```python
from build123d import *

# Parameters (mm, degrees)
HIERRO_ANGULAR_2_X_2_X_0_125_1_DEPTH = 150
CORTAR_EXTRUIR1_DEPTH                = 10
CORTAR_EXTRUIR2_REACH                = 168.317
CROQUIS4_R                           = 2.5


with BuildPart() as part:
    # Sketch1 → Hierro angular 2 X 2 X 0.125(1) (new body)
    with BuildSketch(Plane(origin=(0, 0, 0), x_dir=(1, 0, 0), z_dir=(0, 1, 0))):
        with BuildLine():
            Line((0, 0), (0, 50.8))
            Line((0, 50.8), (0.00508, 50.8))
            ThreePointArc((0.00508, 50.8), (2.246551928, 49.871551928), (3.175, 47.63008))
            Line((3.175, 47.63008), (3.175, 7.9375))
            ThreePointArc((3.175, 7.9375), (4.569903955, 4.569903955), (7.9375, 3.175))
            Line((7.9375, 3.175), (47.63008, 3.175))
            ThreePointArc((47.63008, 3.175), (49.871551928, 2.246551928), (50.8, 0.00508))
            Line((50.8, 0.00508), (50.8, 0))
            Line((50.8, 0), (0, 0))
        make_face()
    extrude(amount=HIERRO_ANGULAR_2_X_2_X_0_125_1_DEPTH)

    # Croquis3 → Cortar-Extruir1 (cut)
    with BuildSketch(Plane.XY):
        Polygon((25, 0), (50.8, 50), (50.8, 0), align=None)
    extrude(amount=-CORTAR_EXTRUIR1_DEPTH, mode=Mode.SUBTRACT)

    # Cortar-Extruir2: up to this face of the body (flat: up to its plane)
    cortar_extruir2_end = Plane(part.part.faces().sort_by_distance((26.665136317, 80.490198143, -3.175))[0])
    # Croquis4 → Cortar-Extruir2 (cut, up to the picked face)
    with BuildSketch(Plane.XY, mode=Mode.PRIVATE) as cortar_extruir2_sk1:
        with Locations((17.9, 140.12)):
            Circle(CROQUIS4_R)
    cortar_extruir2_tool1 = split(extrude(cortar_extruir2_sk1.sketch, amount=-CORTAR_EXTRUIR2_REACH, mode=Mode.PRIVATE), bisect_by=cortar_extruir2_end, keep=Keep.BOTH, mode=Mode.PRIVATE)
    # Croquis4 → Cortar-Extruir2 (cut, up to the picked face)
    with BuildSketch(Plane.XY, mode=Mode.PRIVATE) as cortar_extruir2_sk2:
        with Locations((45.4, 140.12)):
            Circle(CROQUIS4_R)
    cortar_extruir2_tool2 = split(extrude(cortar_extruir2_sk2.sketch, amount=-CORTAR_EXTRUIR2_REACH, mode=Mode.PRIVATE), bisect_by=cortar_extruir2_end, keep=Keep.BOTH, mode=Mode.PRIVATE)
    # Croquis4 → Cortar-Extruir2 (cut, up to the picked face)
    with BuildSketch(Plane.XY, mode=Mode.PRIVATE) as cortar_extruir2_sk3:
        with Locations((17.9, 59.87)):
            Circle(CROQUIS4_R)
    cortar_extruir2_tool3 = split(extrude(cortar_extruir2_sk3.sketch, amount=-CORTAR_EXTRUIR2_REACH, mode=Mode.PRIVATE), bisect_by=cortar_extruir2_end, keep=Keep.BOTH, mode=Mode.PRIVATE)
    # Croquis4 → Cortar-Extruir2 (cut, up to the picked face)
    with BuildSketch(Plane.XY, mode=Mode.PRIVATE) as cortar_extruir2_sk4:
        with Locations((45.4, 59.87)):
            Circle(CROQUIS4_R)
    cortar_extruir2_tool4 = split(extrude(cortar_extruir2_sk4.sketch, amount=-CORTAR_EXTRUIR2_REACH, mode=Mode.PRIVATE), bisect_by=cortar_extruir2_end, keep=Keep.BOTH, mode=Mode.PRIVATE)
    add(cortar_extruir2_tool1.solids().sort_by(Axis((17.9, 140.12, 0), (0, 0, -1)))[0], mode=Mode.SUBTRACT)
    add(cortar_extruir2_tool2.solids().sort_by(Axis((45.4, 140.12, 0), (0, 0, -1)))[0], mode=Mode.SUBTRACT)
    add(cortar_extruir2_tool3.solids().sort_by(Axis((17.9, 59.87, 0), (0, 0, -1)))[0], mode=Mode.SUBTRACT)
    add(cortar_extruir2_tool4.solids().sort_by(Axis((45.4, 59.87, 0), (0, 0, -1)))[0], mode=Mode.SUBTRACT)


solid = part.part
```
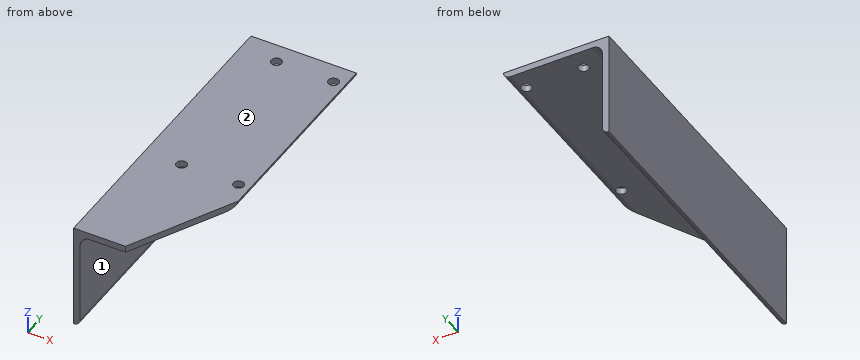
Work out the finished part from the listing and answer in its coordinate system (mm). Face numbers are marked on the shaded views. A direction names the side the tool comes from. Round coordinates to 2 decimals unless told otherwise and drop trailing zeros. Loops run counter-clockwise (first coordinate to the right, second up) from the corner with the lowest first, then second, coordinate; pieces in that order, holes last.
(1) For the marked faces 1 and 2, determine the directions among +Z, -Z, +X, -X, +Y, -Y from which every point of the face is accessible in a straight line to the end or side of a thin tool.
Computed values:
face 1: -Z, +X, +Y, -Y
face 2: +Z, +X, -X, +Y, -Y
(2) The part is cut by section A-A, the plane x = 17.9. Give the vertices of the cut face in (y, z) (3 decimals).
Computed values:
outline: (0, -3.175) - (57.37, -3.175) - (57.37, 0) - (0, 0) - close; (62.37, -3.175) - (137.62, -3.175) - (137.62, 0) - (62.37, 0) - close; (142.62, -3.175) - (150, -3.175) - (150, 0) - (142.62, 0) - close
(3) The part is cut by section D-D, the plane x = 45.4. Give the vertices of the cut face in (y, z) (3 decimals), and give its area (3 significant figures).
Computed values:
outline: (39.535, -3.175) - (57.37, -3.175) - (57.37, 0) - (39.535, 0) - close; (62.37, -3.175) - (137.62, -3.175) - (137.62, 0) - (62.37, 0) - close; (142.62, -3.175) - (150, -3.175) - (150, 0) - (142.62, 0) - close
area: 319 mm2
(4) Each of these flat-tipped pins is pushed along its axis until it touches: P1, Ø12, axis at x = 35, y = 59, coming from the -Z side (3 decimals); P2, Ø5, axis at y = 109, z = -27, coming from the +X side (3 decimals). Where does it stop, or does it pass through?
Computed values:
P1: stops at z = -3.175
P2: stops at x = 3.175
(5) The part is cut by section C-C, the plane z = -29.5. Give the vertices of the cut face in (x, y) (3 decimals).
Computed values:
outline: (0, 0) - (3.175, 0) - (3.175, 150) - (0, 150) - close
(6) Find the intervals of material crossed by L1, parallel to Y at x = 45.4, z = -1.9; L2, parallel to Y at x = 45, z = -1; L3, parallel to X at y = 140, z = -1, in increasing order.
Computed values:
L1: y = 39.53 to 57.37, 62.37 to 137.62, 142.62 to 150
L2: y = 38.76 to 57.4, 62.34 to 137.65, 142.59 to 150
L3: x = 0 to 15.4, 20.4 to 42.9, 47.9 to 50.64
